from build123d import *

# Parameters (mm, degrees)
F0_W     = 12
F0_H     = 27
F0_W_2   = 5
F0_H_2   = 20
F1_DEPTH = 1.2
F3_DEPTH = 4.2
F4_W     = 6.6
F4_H     = 21.6
F5_DEPTH = 0.8


with BuildPart() as f1:
    # F0 (on Front) → F1 (new body)
    with BuildSketch(Plane.XZ):
        Rectangle(F0_W, F0_H)
        Rectangle(F0_W_2, F0_H_2, mode=Mode.SUBTRACT)
    extrude(amount=F1_DEPTH)

    # F2 (on face) → F3 (join)
    with BuildSketch(Plane.XZ.offset(1.2)):
        Polygon((-2.5, -10.8), (-2.5, 10), (2.5, 10), (2.5, -10), (2.5, -10.8), (3.3, -10.8), (3.3, 10.8), (-3.3, 10.8), (-3.3, -10.8), align=None)
    extrude(amount=F3_DEPTH)

    # F4 (on face) → F5 (join)
    with BuildSketch(Plane.XZ.offset(5.4)):
        Rectangle(F4_W, F4_H)
    extrude(amount=F5_DEPTH)


solid = f1.part
For this review, take the finished solid that the model builds, in its own axes (mm). A direction names the side the tool comes from. Coordinates: 2 decimals unless noted, no trailing zeros. Write each loop counter-clockwise with the first axis right and the second up, starting at its lowest first coordinate (ties: lowest second). Pieces come first, ordered by that corner, then holes. Notation, with made-up numbers: (-38.75, -3) -> (19.25, -3) arc R23 cw to (19.25, 29) -> close; hole circle Ø6 at (65, -26.5). An arc over 180 degrees is marked (long way). Write each question's results on one line, items separated by ' | '. Start each with the question number.
1) Consider section A-A (x = -0.75). Write out the cut boundary in (y, z), plus the area to 3 significant figures.
2) Consider section D-D (z = -9). Write out the cut boundary in (x, y).
3) Wall thickness on L1, parallel to X at y = -3.75, z = -1.5; L2, parallel to Z at x = 0.75, y = -1; L3, parallel to X at y = -1, z = -4.25: over which ranges is each line inside the solid? List them lowest first. Write a range as [from, to].
4) Consider section B-B (y = -0.5). Write out the cut boundary in (x, z), plus the area to 3 significant figures.
5) The part is to be moulded in two halves that separate along X. For faces 1 (the face through (0, -3, 10)), 2 (the face through (0, -6, -10.8)), 3 (the face through (6, -1, 0)), say which applies: +X half, -X half, draft (parallel to the pull), parting line (faces both ways), or undercut.
6) For faces 4 (the face through (3.3, -4, 0)), 5 (the face through (-3.3, -4, 0)), 6 (the face through (0, -1, -10)), 7 (the face through (0, -4, 10.8)), list the 3-axis set-ups (+Z, -Z, +X, -X, +Y, -Y) from which the entire face can be reached by the end or side of a thin tool; tool diameter is ignored.
7) Consider section C-C (y = -1.75). Write out the cut boundary in (x, z), plus the area to 3 significant figures.
8) Insertion check: pin 1 (2.5 mm diameter, centred on x = -0.5, y = -4, fed in from -Z); pin 2 (2.5 mm diameter, centred on y = -3, z = 0, fed in from +X); pin 3 (1 mm diameter, centred on x = 2, y = -2, fed in from +Z). Each pin has a flat end and moves straight along its axis. Give the tip position at first contact, or say it passes through.
Geometry says:
1) outline: (-6.2, -10.8) -> (-5.4, -10.8) -> (-5.4, 10) -> (0, 10) -> (0, 13.5) -> (-1.2, 13.5) -> (-1.2, 10.8) -> (-6.2, 10.8) -> close; (-1.2, -13.5) -> (0, -13.5) -> (0, -10) -> (-1.2, -10) -> close | area: 29.0 mm^2
2) outline: (-6, -1.2) -> (-3.3, -1.2) -> (-3.3, -6.2) -> (3.3, -6.2) -> (3.3, -1.2) -> (6, -1.2) -> (6, 0) -> (2.5, 0) -> (2.5, -5.4) -> (-2.5, -5.4) -> (-2.5, 0) -> (-6, 0) -> close
3) L1: [-3.3, -2.5], [2.5, 3.3] | L2: [-13.5, -10], [10, 13.5] | L3: [-6, -2.5], [2.5, 6]
4) outline: (-6, -13.5) -> (6, -13.5) -> (6, 13.5) -> (-6, 13.5) -> close; hole (-2.5, -10) -> (2.5, -10) -> (2.5, 10) -> (-2.5, 10) -> close | area: 224 mm^2
5) face 1: undercut | face 2: draft | face 3: +X half
6) face 4: +Z, -Z, +X, -Y | face 5: +Z, -Z, -X, -Y | face 6: +Y | face 7: +Z, +X, -X, -Y
7) outline: (-3.3, -10.8) -> (-2.5, -10.8) -> (-2.5, 10) -> (2.5, 10) -> (2.5, -10.8) -> (3.3, -10.8) -> (3.3, 10.8) -> (-3.3, 10.8) -> close | area: 38.6 mm^2
8) pin 1: z = 10 | pin 2: x = 3.3 | pin 3: z = 10.8
